Here's how the part is built. I have some questions about the finished solid (model axes, mm). A direction names the side the tool comes from. Round coordinates to 2 decimals unless told otherwise and drop trailing zeros. Loops run counter-clockwise (first coordinate to the right, second up) from the corner with the lowest first, then second, coordinate; pieces in that order, holes last. Notation, with made-up numbers: M 28.5,17.25 L 63.5,17.25 A20 cw 63.5,45.25 Z; hole C 52,64.5 d5. An arc over 180 degrees is marked long. Answer as CSV lines item,"result".
```python
from build123d import *

# Parameters (mm, degrees)
SKETCH1_R           = 2.1
BOSS_EXTRUDE1_DEPTH = 3
SKETCH2_R           = 2.1
BOSS_EXTRUDE2_DEPTH = 3
FILLET1_R           = 2


with BuildPart() as part:
    # Sketch1 → Boss-Extrude1 (new body)
    with BuildSketch(Plane(origin=(0, 0, 0), x_dir=(1, 0, 0), z_dir=(0, 1, 0))):
        Polygon((-6, 0), (6, 0), (6, -57), (-17, -57), (-17, -33), (-6, -33), align=None)
        with Locations((-11.9, -37)):
            Circle(SKETCH1_R, mode=Mode.SUBTRACT)
        with Locations((-11.9, -53)):
            Circle(SKETCH1_R, mode=Mode.SUBTRACT)
    extrude(amount=BOSS_EXTRUDE1_DEPTH)

    # Sketch2 → Boss-Extrude2 (add)
    with BuildSketch(Plane.XY):
        Polygon((6, 0), (-6, 0), (-6, 43.9), (-24, 43.9), (-24, 52.1), (6, 52.1), align=None)
        with Locations((-19.9, 48)):
            Circle(SKETCH2_R, mode=Mode.SUBTRACT)
        with Locations((-3.9, 48)):
            Circle(SKETCH2_R, mode=Mode.SUBTRACT)
    extrude(amount=-BOSS_EXTRUDE2_DEPTH)

    # Fillet1
    fillet1_edges = [part.edges().sort_by_distance(p)[0] for p in [
        (6, 1.5, 57),
        (-17, 1.5, 57),
        (-17, 1.5, 33),
        (-6, 1.5, 33),
        (6, 52.1, -1.5),
        (-6, 43.9, -1.5),
        (-24, 43.9, -1.5),
        (-24, 52.1, -1.5),
    ]]
    fillet(fillet1_edges, radius=FILLET1_R)


solid = part.part
```
1. I want a section at C-C, the plane y = 48. Please give me the cut outline in (x, z).
Evaluation:
outline,"M -24,-3 L -22,-3 L -22,0 L -24,0 Z; M -17.8,-3 L -6,-3 L -6,0 L -17.8,0 Z; M -1.8,-3 L 6,-3 L 6,0 L -1.8,0 Z"
2. I want a section at A-A, the plane z = 37. Please give me the cut outline in (x, y), and give its area (3 significant figures).
Evaluation:
outline,"M -17,0 L -14,0 L -14,3 L -17,3 Z; M -9.8,0 L 6,0 L 6,3 L -9.8,3 Z"
area,"56.4 mm²"
3. I want a section at B-B, the plane x = -3.9. Please give me the cut outline in (y, z), and give its area (3 significant figures).
Evaluation:
outline,"M 0,-3 L 45.9,-3 L 45.9,0 L 3,0 L 3,57 L 0,57 Z; M 50.1,-3 L 52.1,-3 L 52.1,0 L 50.1,0 Z"
area,"315 mm²"
4. We'd pull the mould along Y, two halves only. Please class faces 1 (the cylindrical face through (-23.43, 51.5, -1.52)), 2 (the cylindrical face through (-18.931, 46.137, -1.479)), 3 (the flat face through (-2, 26, -3)): pulls with the +Y half, pulls with the -Y half, needs draft (parallel to the pull), parting line crosses it, or undercut.
Evaluation:
face 1,"pulls with the +Y half"
face 2,"undercut"
face 3,"needs draft"
5. If I drill on line 1 (Z direction, x = -11.9, y = 1.8); line 2 (X direction, y = 2, z = 37); line 3 (Y direction, x = -3.9, z = -2), over which ranges is the centre line in solid material (lowest first)? Write a range as [from, to].
Evaluation:
line 1,"z = [33, 34.9], [39.1, 50.9], [55.1, 57]"
line 2,"x = [-17, -14], [-9.8, 6]"
line 3,"y = [0, 45.9], [50.1, 52.1]"
6. For P1, Ø2.5, axis at x = -11.9, z = 37, coming from the +Y side; P2, Ø3, axis at x = -7, y = 5.5, coming from the +Z side; P3, Ø2.5, axis at x = -10.5, y = 2, coming from the -Z side; P4, Ø3.5, axis at y = 1, z = 47, coming from the -X side, each with a flat end and sliding along its axis, tell me the tip position at first contact or that it passes through.
Evaluation:
P1,"passes through"
P2,"stops at z = 0"
P3,"stops at z = 33"
P4,"stops at x = -17"
7. I want a section at D-D, the plane x = -11.9. Please give me the cut outline in (y, z), and give its area (3 significant figures).
Evaluation:
outline,"M 0,33 L 3,33 L 3,34.9 L 0,34.9 Z; M 0,39.1 L 3,39.1 L 3,50.9 L 0,50.9 Z; M 0,55.1 L 3,55.1 L 3,57 L 0,57 Z; M 43.9,-3 L 52.1,-3 L 52.1,0 L 43.9,0 Z"
area,"71.4 mm²"
8. Which directions (+Z, -Z, +X, -X, +Y, -Y) give clear straight access to the entire face, cutting with the end or side of a thin tool? Please do faces 4 (the flat face through (-12, 1, 33)), 5 (the flat face through (-3, 3, 34)), 6 (the cylindrical face through (5.4, 1.52, 56.43)), 7 (the flat face through (-15, 43.9, -1)), 8 (the flat face through (-17, 1, 45)).
Evaluation:
face 4,"-Z, -X, +Y, -Y"
face 5,"+Z, +X, -X, +Y"
face 6,"+Z, +X, +Y, -Y"
face 7,"+Z, -Z, -X, -Y"
face 8,"+Z, -Z, -X, +Y, -Y"
